Part print with two shaded views. Sizes in mm from the minimum x, y, z corner. Give positions to 0.01 mm unless a question says otherwise; leave off trailing zeros. Loops run counter-clockwise (first coordinate to the right, second up) from the corner with the lowest first, then second, coordinate; pieces in that order, holes last. Notation, with made-up numbers: (74, -19.75) -> (79, -19.75) arc R18 cw to (79, 1.25) -> close; hole circle Ø7 at (15, 75.25). An arc over 180 degrees is marked (long way). One line per question, with ' | ' between items. Start each with the question number.
(1) Flat gauge pins, fed straight in: pin 1 Ø1 at (x, y) = (11.5, 2) entering from -Z; pin 2 Ø1 at (x, z) = (11, 2) entering from -Y. Where does each tip first touch, or does it go through?
(2) Mould opens along X. For the marked faces 1, 2 and 3 say: pulls with the +X half, pulls with the -X half, needs draft (parallel to the pull), parting line crosses it, or undercut.
(3) Slice it at A-A, the plane y = 0.85. Write the cut outline in (x, z).
(4) Drill centre lines: L1, parallel to X at y = 2.4, z = 7; L2, parallel to Z at x = 7.5, y = 2.85; L3, parallel to X at y = 1.9, z = 9.75. Where is each one in solid material? Low to high. Write a range as from..to.
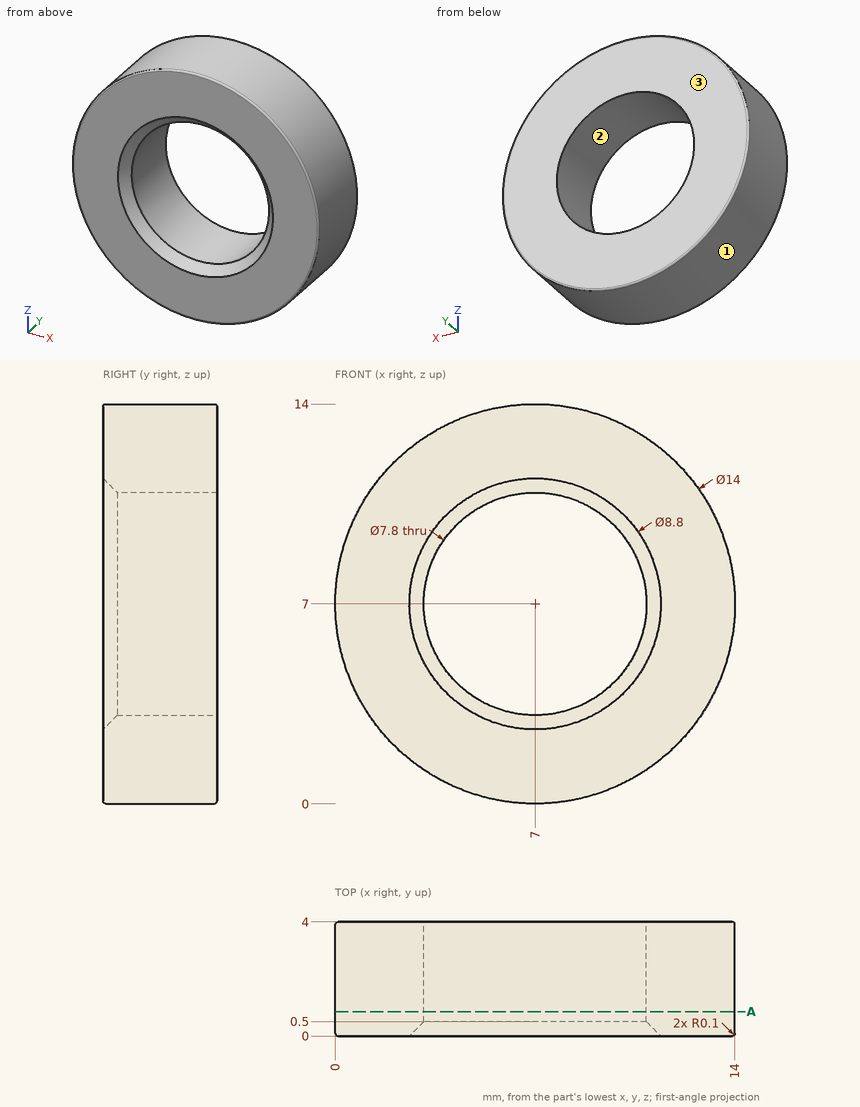
Final values:
1) pin 1: z = 1.26 | pin 2: y = 0
2) face 1: parting line crosses it | face 2: undercut | face 3: needs draft
3) outline: circle Ø14 at (7, 7); hole circle Ø7.8 at (7, 7)
4) L1: 0..3.1, 10.9..14 | L2: 0.02..3.13, 10.87..13.98 | L3: 0.56..4.23, 9.77..13.44
